Input: dimensioned drawing with shaded views. Units: mm. Origin: part minimum x, y, z. Coordinates: 2 decimals unless noted, no trailing zeros. Loops run counter-clockwise (first coordinate to the right, second up) from the corner with the lowest first, then second, coordinate; pieces in that order, holes last. Notation, with made-up numbers: M -26.75,10.25 L 7.25,10.25 A23 ccw 7.25,26.25 Z; hole C 46,32 d8. An arc over 180 degrees is marked long. Write item = value, one per line. Start each with the question number.
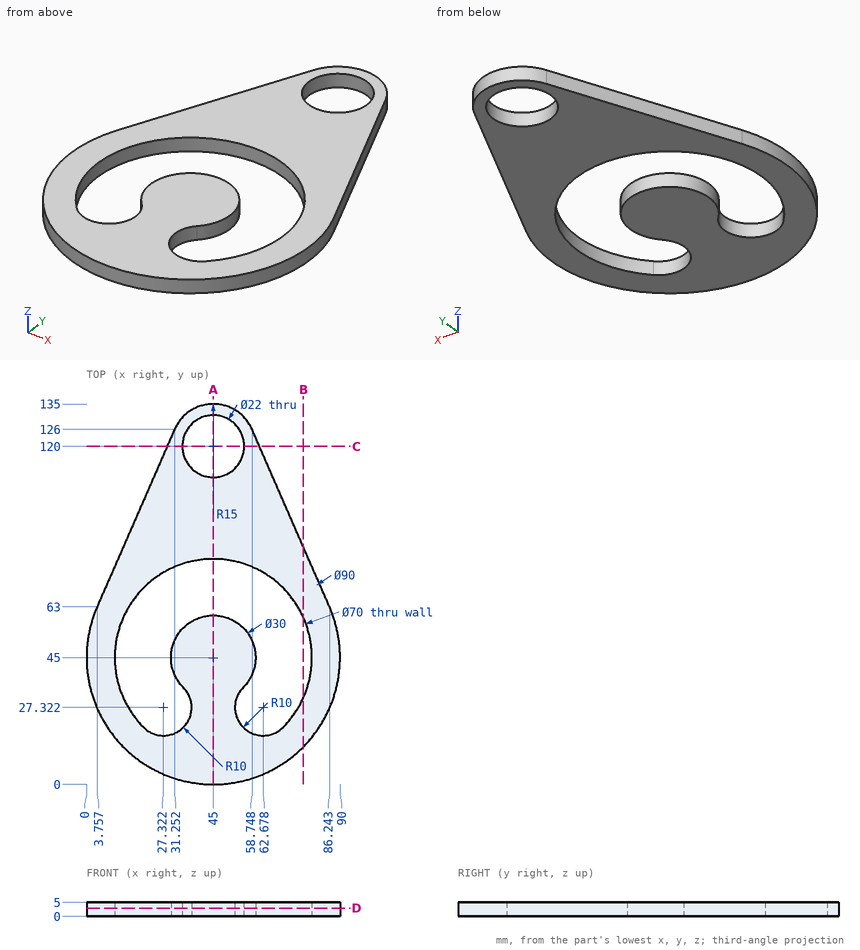
Item 1: Section query D-D (z = 3). Return the cut outline in (x, y), plus the area to 3 significant figures.
Item 2: Section query C-C (y = 120). Return the cut outline in (x, z).
Item 3: Section query B-B (x = 77). Return the cut outline in (y, z).
Item 4: Line query: line 1 (X direction, y = 45, z = 1); line 2 (X direction, y = 50, z = 3.65); line 3 (Y direction, x = 44, z = 1.85) (1 decimal). Output: solid intervals per line, ascending. Write a range as from..to.
Item 5: First-contact query: pin 1 (1 mm diameter, centred on x = 46.5, z = 3.5, fed in from +Y); pin 2 (1 mm diameter, centred on x = 67, z = 4.5, fed in from +Y) (1 decimal); pin 3 (1.5 mm diameter, centred on y = 41.5, z = 2, fed in from +X); pin 4 (12 mm diameter, centred on x = 16.5, y = 47, fed in from -Z). Flat tips, straight axial feed; report the tip coordinate or a pass-through.
Item 6: Section query A-A (x = 45). Return the cut outline in (y, z).
Verdict:
q1.outline = M 3.76,63 A45 ccw long 86.24,63 L 58.75,126 A15 ccw 31.25,126 Z; hole M 20.25,20.25 A10 ccw 34.39,34.39 A15 cw long 55.61,34.39 A10 ccw 69.75,20.25 A35 ccw long Z; hole C 45,120 d22
q1.area = 5,350 mm2
q2.outline = M 28.63,0 L 34,0 L 34,5 L 28.63,5 Z; M 56,0 L 61.37,0 L 61.37,5 L 56,5 Z
q3.outline = M 13.36,0 L 30.82,0 L 30.82,5 L 13.36,5 Z; M 59.18,0 L 84.18,0 L 84.18,5 L 59.18,5 Z
q4.line_1 = 0..10, 30..60, 80..90
q4.line_2 = 0.28..10.36, 30.86..59.14, 79.64..89.72
q4.line_3 = 0..60, 80..109, 131..135
q5.pin_1 = 134.97
q5.pin_2 = 108.2
q5.pin_3 = 89.92
q5.pin_4 = through
q6.outline = M 0,0 L 60,0 L 60,5 L 0,5 Z; M 80,0 L 109,0 L 109,5 L 80,5 Z; M 131,0 L 135,0 L 135,5 L 131,5 Z
